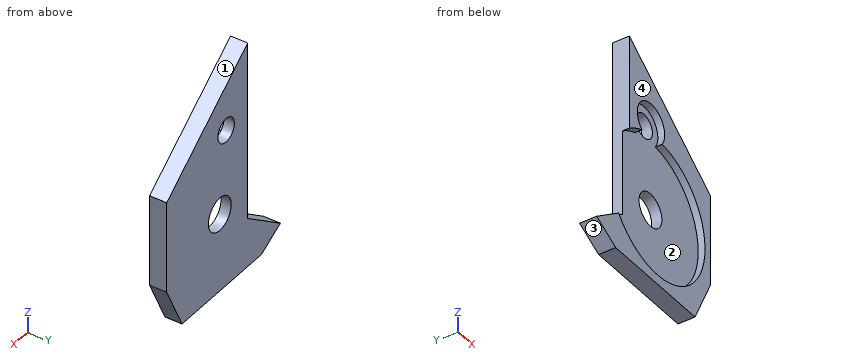
```python
from build123d import *

# Parameters (mm, degrees)
EXTRUDE_1_DEPTH     = 5
CUT_EXTRUDE_1_DEPTH = 2
SKETCH_3_R          = 4.87
SKETCH_3_R_2        = 3.5
CUT_EXTRUDE_2_DEPTH = 80.472580045


with BuildPart() as part:
    # Эскиз1 → Вытянуть1 (new body)
    with BuildSketch(Plane(origin=(0, 0, 0), x_dir=(1, 0, 0), z_dir=(0, 1, 0))):
        Polygon((1e-09, -1e-09), (8.096990259, 4.437064442), (41.925316116, 4.437064442), (48.461562516, -9.134468652), (48.461562516, -36.044162995), (13.950964491, -62.788278664), (13.949330464, -10.03402267), align=None)
    extrude(amount=EXTRUDE_1_DEPTH)

    # Эскиз2 → Вырез-Вытянуть1 (cut)
    with BuildSketch(Plane.XZ):
        with BuildLine():
            ThreePointArc((19.270119717, 37.867537317), (28.134312971, -1.551588069), (27.906130369, 38.851249714))
            ThreePointArc((27.906130369, 38.851249714), (22.488439096, 48.013535902), (19.270119717, 37.867537317))
        make_face()
    extrude(amount=-CUT_EXTRUDE_1_DEPTH, mode=Mode.SUBTRACT)

    # Эскиз3 → Вырез-Вытянуть2 (cut, through all)
    with BuildSketch(Plane(origin=(0, 5, 0), x_dir=(1, 0, 0), z_dir=(0, 1, 0))):
        with Locations(Location((25.834611823, -18.637487181, 0), (0, 0, 270))):
            Circle(SKETCH_3_R)
        with Locations(Location((23.148278256, -42.220808245, 0), (0, 0, 270))):
            Circle(SKETCH_3_R_2)
    extrude(amount=-CUT_EXTRUDE_2_DEPTH, mode=Mode.SUBTRACT)


solid = part.part
```
Here's how the part is built. I have some questions about the finished solid (model axes, mm). Face numbers are marked on the shaded views. Round coordinates to 2 decimals unless told otherwise and drop trailing zeros. Write each loop counter-clockwise with the first axis right and the second up, starting at its lowest first coordinate (ties: lowest second). Pieces come first, ordered by that corner, then holes. Notation, with made-up numbers: M -38.75,31 L 15.25,31 A14 cw 15.25,50 Z; hole C 87,74 d8. An arc over 180 degrees is marked long. Answer as CSV lines item,"result". Start each with the question number.
1. I need wall thicknesses on probe 1 along Z at (x, y) = (25, 3.4); probe 2 along Y at (x, z) = (23, 33); probe 3 along Z at (x, y) = (38, 1.25). Which ranges of each line are inside material? Lowest first, please.
2. Thinking about a two-plate mould opening in X: for the marked faces 1, 2, 3 and 4, which applies, released by +X, released by -X, zero draft, split by the parting line, or undercut?
3. Suppose I cut it at D-D on x = 43. Write out the boundary of the cut face in (y, z).
4. Suppose I cut it at A-A on x = 24. Write out the boundary of the cut face in (y, z), then the cut area to 3 significant figures.
5. Suppose I cut it at B-B on z = 43. Write out the boundary of the cut face in (x, y).
6. I'm going to push flat-ended pins straight in: pin 1 Ø1 at (x, y) = (35.5, 2.5) entering from +Z; pin 2 Ø3 at (y, z) = (2, 56) entering from +X; pin 3 Ø9 at (x, z) = (23.15, 42.22) entering from +Y; pin 4 Ø9.5 at (x, z) = (23.15, 42.22) entering from -Y. Where does each tip first touch, or does it pass through?
7. Suppose I cut it at C-C on y = 3.05. Write out the boundary of the cut face in (x, z), then the cut area to 3 significant figures.
Check result:
1,probe 1,"z = -4.44 to 13.84, 23.44 to 39.25, 45.19 to 54.23"
1,probe 2,"y = 2 to 5"
1,probe 3,"z = -4.44 to 2.36, 34.91 to 44.15"
2,face 1,"released by +X"
2,face 2,"undercut"
2,face 3,"released by -X"
2,face 4,"zero draft"
3,outline,"M 0,-2.21 L 5,-2.21 L 5,40.28 L 0,40.28 L 0,29.51 L 2,29.51 L 2,7.76 L 0,7.76 Z"
4,outline,"M 0,-4.44 L 5,-4.44 L 5,14.13 L 2,14.13 L 2,-1.6 L 0,-1.6 Z; M 0,47.99 L 2,47.99 L 2,45.62 L 5,45.62 L 5,55 L 0,55 Z; M 2,23.15 L 5,23.15 L 5,38.83 L 2,38.83 Z"
4,area,"151 mm2"
5,outline,"M 13.95,0 L 17.37,0 L 17.37,2 L 19.74,2 L 19.74,5 L 13.95,5 Z; M 26.56,2 L 28.93,2 L 28.93,0 L 39.49,0 L 39.49,5 L 26.56,5 Z"
6,pin 1,"stops at z = 46.48"
6,pin 2,"stops at x = 24.65"
6,pin 3,"stops at y = 5"
6,pin 4,"stops at y = 2"
7,outline,"M 0,0 L 8.1,-4.44 L 41.93,-4.44 L 48.46,9.13 L 48.46,36.04 L 13.95,62.79 L 13.95,10.03 Z; hole C 23.15,42.22 d7; hole C 25.83,18.64 d9.74"
7,area,"1,820 mm2"
